For this review, use the dimensioned drawing (mm, ordinates from the lowest corner) and the shaded views. A direction names the side the tool comes from. Round coordinates to 2 decimals unless told otherwise and drop trailing zeros. Write each loop counter-clockwise with the first axis right and the second up, starting at its lowest first coordinate (ties: lowest second). Pieces come first, ordered by that corner, then holes. Notation, with made-up numbers: M 72,-37 L 89,-37 A5 ccw 89,-32 Z; hole C -13,-7 d5. An arc over 180 degrees is marked long. One line per question, with ' | ' between items. Start each with the question number.
Item 1: Add section B-B, the plane y = 22.5. State the section outline as (x, z) points.
Item 2: For L1, parallel to Y at x = 21, z = 27.5; L2, parallel to X at y = 13.5, z = 44.5; L3, parallel to X at y = 15, z = 27.5 (1 decimal), list the stretches that pass through material, from the lowest coordinate up.
Item 3: Add section C-C, the plane z = 10. State the section outline as (x, y) points, and give its area (3 significant figures).
Item 4: Add section D-D, the plane y = 4.5. State the section outline as (x, z) points.
Item 5: Add section A-A, the plane x = 21. State the section outline as (y, z) points.
Item 6: Insertion check: pin 1 Ø6 at (x, z) = (8.5, 36) entering from +Y; pin 2 Ø2 at (y, z) = (40.5, 20) entering from +X; pin 3 Ø5 at (x, z) = (26, 13.5) entering from -Y. Each pin has a flat end and moves straight along its axis. Give the tip position at first contact, or say it passes through.
Item 7: Draft analysis for pull direction X (two halves, no side actions). For the marked faces 4, 5 and 6, state which applies: released by +X, released by -X, zero draft, split by the parting line, or undercut.
Item 8: Machinability: for the marked faces 1, 2 and 3, which of the approach directions +Z, -Z, +X, -X, +Y, -Y give a long, thin tool a straight path to every point of the face, cutting with its end or side? Answer none if there is none.
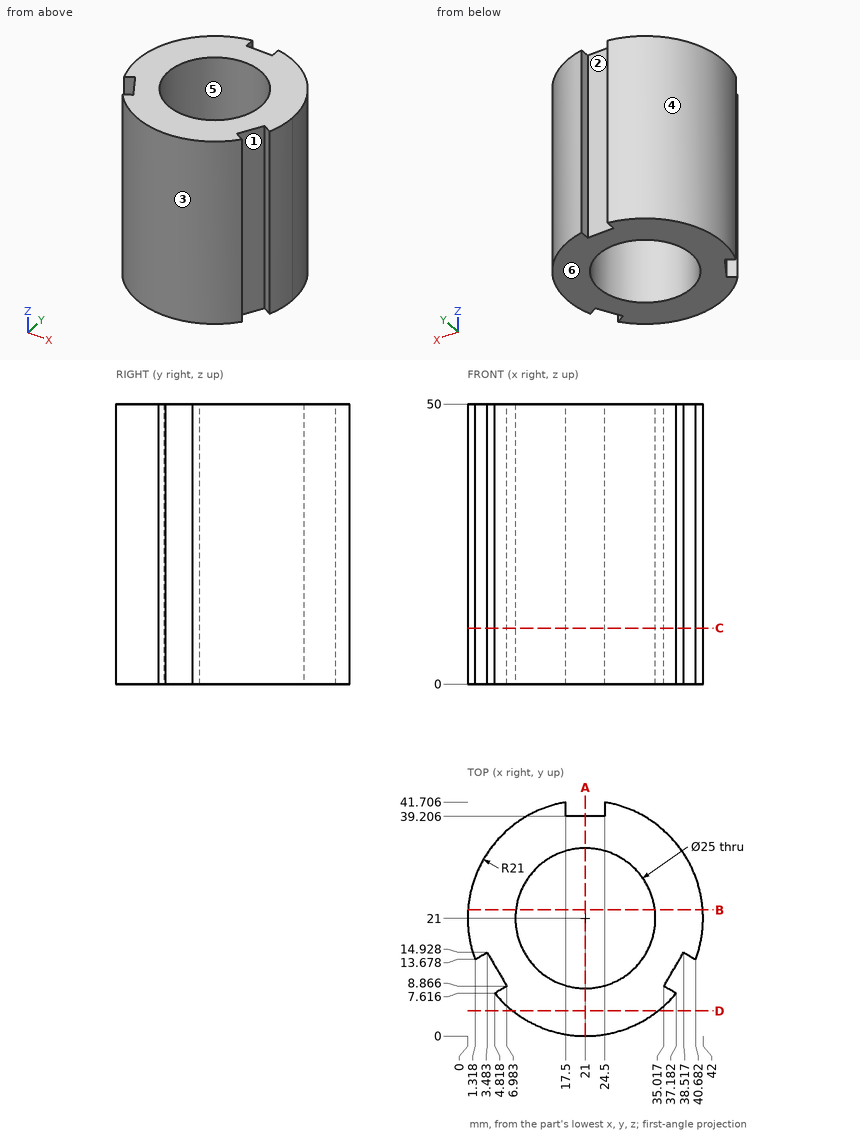
Computed values:
1) outline: M 0.05,0 L 8.59,0 L 8.59,50 L 0.05,50 Z; M 33.41,0 L 41.95,0 L 41.95,50 L 33.41,50 Z
2) L1: y = 0 to 8.5, 33.5 to 39.21 | L2: x = 4.31 to 11, 31 to 37.69 | L3: x = 0.9 to 10, 32 to 41.1
3) outline: M 1.32,13.68 L 3.48,14.93 L 6.98,8.87 L 4.82,7.62 A21 ccw 37.18,7.62 L 35.02,8.87 L 38.52,14.93 L 40.68,13.68 A21 ccw 24.5,41.71 L 24.5,39.21 L 17.5,39.21 L 17.5,41.71 A21 ccw Z; hole C 21,21 d25 | area: 838 mm^2
4) outline: M 8.01,0 L 33.99,0 L 33.99,50 L 8.01,50 Z
5) outline: M 0,0 L 8.5,0 L 8.5,50 L 0,50 Z; M 33.5,0 L 39.21,0 L 39.21,50 L 33.5,50 Z
6) pin 1: stops at y = 39.73 | pin 2: stops at x = 30.94 | pin 3: stops at y = 0.15
7) face 4: released by -X | face 5: undercut | face 6: zero draft
8) face 1: +Z, -Z | face 2: +Z, -Z, +Y | face 3: +Z, -Z, -Y
